```python
from build123d import *

# Parameters (mm, degrees)
ESQUISSE1_R                               = 10
BOSS_EXTRU_1_DEPTH                        = 10
D_GAGEMENT_M41_D                          = 4.3
D_GAGEMENT_M41_DEPTH                      = 8
D_GAGEMENT_M41_TIP                        = 1.291850331
ESQUISSE4_R                               = 27.5
BOSS_EXTRU_2_DEPTH                        = 10
ESQUISSE5_R                               = 10
BOSS_EXTRU_3_DEPTH                        = 2
TROU_POUR_TARAUDAGE_POUR_TROU_TARAUD_M5_D = 4.2
R_P_TITION_CIRCULAIRE1_COUNT              = 4
CHANFREIN1_SIZE                           = 0.5
CHANFREIN2_SIZE                           = 0.2


with BuildPart() as part:
    # Esquisse1 → Boss.-Extru.1 (new body)
    with BuildSketch(Plane(origin=(0, 0, 0), x_dir=(1, 0, 0), z_dir=(0, 1, 0))):
        with Locations(Location((0, 0, 0), (0, 0, 270))):
            Circle(ESQUISSE1_R)
        with BuildLine():
            Line((-1.936491673, 3.5), (1.936491673, 3.5))
            ThreePointArc((1.936491673, 3.5), (0, -4), (-1.936491673, 3.5))
        make_face(mode=Mode.SUBTRACT)
    extrude(amount=BOSS_EXTRU_1_DEPTH)

    # D_gagement M41
    with Locations(Plane(origin=(0, 0, -10), x_dir=(-1, 0, 0), z_dir=(0, 0, -1))):
        with Locations((0, 5)):
            Hole(D_GAGEMENT_M41_D / 2, depth=D_GAGEMENT_M41_DEPTH)
            with Locations((0, 0, -(D_GAGEMENT_M41_DEPTH + D_GAGEMENT_M41_TIP / 2))):  # 118° drill point
                Cone(0, D_GAGEMENT_M41_D / 2, D_GAGEMENT_M41_TIP, mode=Mode.SUBTRACT)

    # Esquisse4 → Boss.-Extru.2 (add)
    with BuildSketch(Plane(origin=(0, 10, 0), x_dir=(1, 0, 0), z_dir=(0, 1, 0))):
        with Locations(Location((0, 0, 0), (0, 0, 270))):
            Circle(ESQUISSE4_R)
        with BuildLine():
            Line((-1.936491673, 3.5), (1.936491673, 3.5))
            ThreePointArc((1.936491673, 3.5), (0, -4), (-1.936491673, 3.5))
        make_face(mode=Mode.SUBTRACT)
    extrude(amount=BOSS_EXTRU_2_DEPTH)

    # Esquisse5 → Boss.-Extru.3 (add)
    with BuildSketch(Plane(origin=(0, 20, 0), x_dir=(1, 0, 0), z_dir=(0, 1, 0))):
        with Locations(Location((0, 0, 0), (0, 0, 270))):
            Circle(ESQUISSE5_R)
        with BuildLine():
            Line((-1.936491673, 3.5), (1.936491673, 3.5))
            ThreePointArc((1.936491673, 3.5), (0, -4), (-1.936491673, 3.5))
        make_face(mode=Mode.SUBTRACT)
    extrude(amount=BOSS_EXTRU_3_DEPTH)

    # Trou pour taraudage pour trou taraud_ M5 (through all)
    with Locations(Plane(origin=(0, 20, 0), x_dir=(1, 0, 0), z_dir=(0, 1, 0))):
        with Locations((0, -20)):
            trou_pour_taraudage_pour_trou_taraud_m5 = Hole(TROU_POUR_TARAUDAGE_POUR_TROU_TARAUD_M5_D / 2)

    # R_p_tition circulaire1: Trou pour taraudage pour trou taraud_ M5 ×4 about axis
    r_p_tition_circulaire1_axis = Axis((0, 0, 0), (0, 1, 0))
    for i in range(1, R_P_TITION_CIRCULAIRE1_COUNT):
        add(trou_pour_taraudage_pour_trou_taraud_m5.rotate(r_p_tition_circulaire1_axis, i * 360 / R_P_TITION_CIRCULAIRE1_COUNT), mode=Mode.SUBTRACT)

    # Chanfrein1
    chanfrein1_edges = [part.edges().sort_by_distance(p)[0] for p in [
        (0, 0, -10),
        (0, 20, -27.5),
        (0, 10, -27.5),
    ]]
    chamfer(chanfrein1_edges, length=CHANFREIN1_SIZE)

    # Chanfrein2
    chanfrein2_edges = [part.edges().sort_by_distance(p)[0] for p in [
        (0, 22, -10),
    ]]
    chamfer(chanfrein2_edges, length=CHANFREIN2_SIZE)


solid = part.part
```
Could you check a few things on this model? Use its own coordinates, in mm. A direction names the side the tool comes from. Give positions to 0.01 mm unless a question says otherwise; leave off trailing zeros. Order: outer loops, then holes, each group sorted by start corner. A loop starts at its lowest first (then second) coordinate and runs counter-clockwise, first axis right, second up.
Q1. Suppose I cut it at A-A, the plane y = 14. Write out the boundary of the cut face in (x, z), and give its area (3 significant figures).
Q2. For faces 1 (the cylindrical face through (3, 5.18, 9.54)), 2 (the flat face through (0, 2, -3.5)), 3 (the flat face through (-4, 0, 2)), 4 (the cylindrical face through (-9.76, 20.89, -2.17)), which set-ups out of +Z, -Z, +X, -X, +Y, -Y let a thin tool reach every point of the face, with its end or its side?
Q3. We'd pull the mould along Z, two halves only. Please class faces 5 (the flat face through (0, 20, 12)), 6 (the cylindrical face through (-24.397, 14.937, 12.69)), 7 (the cylindrical face through (0, 11, 4)): +Z half, -Z half, draft (parallel to the pull), parting line (faces both ways), or undercut.
Q4. Suppose I cut it at C-C, the plane y = 1.75. Write out the boundary of the cut face in (x, z).
Q5. If I drill on line 1 along X through (y, z) = (17.25, 0); line 2 along X through (y, z) = (5.5, 0); line 3 along Y through (x, z) = (0, -8.25), over which ranges is the centre line in solid material (lowest first)?
Q6. I'm going to push flat-ended pins straight in: P1, Ø6, axis at x = -5.5, y = 8, coming from the -Z side; P2, Ø8, axis at y = 6.5, z = 21, coming from the -X side; P3, Ø3.5, axis at x = 0, y = 5, coming from the -Z side. Where does each tip first touch, or does it pass through?
Q7. Suppose I cut it at D-D, the plane y = 5. Write out the boundary of the cut face in (x, z).
Q8. Suppose I cut it at B-B, the plane z = 0. Count the separate pieces of the cut face and the enclosed holes in it, and give its area (3 significant figures).
Solution:
1. outline: circle Ø55 at (0, 0); hole circle Ø4.2 at (-20, 0); hole circle Ø4.2 at (0, -20); hole circle Ø4.2 at (0, 20); hole (-1.94, -3.5) - (1.94, -3.5) arc R4 ccw (long way) to start; hole circle Ø4.2 at (20, 0)
1. area: 2,270 mm2
2. face 1: -Y
2. face 2: +Y, -Y
2. face 3: +Z, -Z, +X, -X, -Y
2. face 4: +Y
3. face 5: draft
3. face 6: parting line
3. face 7: undercut
4. outline: circle Ø20 at (0, 0); hole (-1.94, -3.5) - (1.94, -3.5) arc R4 ccw (long way) to start
5. line 1: x = -27.5 to -22.1, -17.9 to -4, 4 to 17.9, 22.1 to 27.5
5. line 2: x = -10 to -4, 4 to 10
5. line 3: y = 0 to 2.85, 7.15 to 22
6. P1: stops at z = -27.23
6. P2: stops at x = -19.12
6. P3: stops at z = 3.6
7. outline: (-2.15, -9.77) - (-2.15, -3.37) arc R4 cw (long way) to (2.15, -3.37) - (2.15, -9.77) arc R10 ccw (long way) to start
8. separate pieces: 4
8. enclosed holes: 0
8. area: 529 mm2
